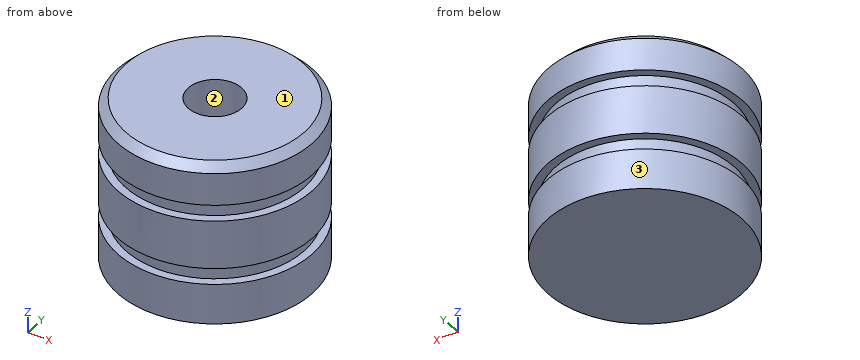
```python
from build123d import *

# Parameters (mm, degrees)
SKETCH1_R                 = 6
BOSS_EXTRUDE1_DEPTH       = 5
CUT_EXTRUDE1_START        = -2.5
SKETCH2_R                 = 6
SKETCH2_R_2               = 5.5
CUT_EXTRUDE1_DEPTH        = 1
CHAMFER1_SIZE             = 0.5
M4X0_7_TAPPED_HOLE1_D     = 3.3
M4X0_7_TAPPED_HOLE1_DEPTH = 8
M4X0_7_TAPPED_HOLE1_TIP   = 0.991420021


with BuildPart() as part:
    # Sketch1 → Boss-Extrude1 (new body, symmetric)
    with BuildSketch(Plane.XY):
        Circle(SKETCH1_R)
    extrude(amount=BOSS_EXTRUDE1_DEPTH, both=True)

    # Sketch2 → Cut-Extrude1 (cut)
    with BuildSketch(Plane.XY.offset(5).offset(CUT_EXTRUDE1_START)):
        Circle(SKETCH2_R)
        Circle(SKETCH2_R_2, mode=Mode.SUBTRACT)
    cut_extrude1 = extrude(amount=-CUT_EXTRUDE1_DEPTH, mode=Mode.SUBTRACT)

    # Mirror1: Cut-Extrude1 across plane
    add(cut_extrude1.mirror(Plane.XY), mode=Mode.SUBTRACT)

    # Chamfer1
    chamfer1_edges = [part.edges().sort_by_distance(p)[0] for p in [
        (-6, 0, 5),
    ]]
    chamfer(chamfer1_edges, length=CHAMFER1_SIZE)

    # M4x0.7 Tapped Hole1
    with Locations(Plane.XY.offset(5)):
        with Locations((0, 0)):
            Hole(M4X0_7_TAPPED_HOLE1_D / 2, depth=M4X0_7_TAPPED_HOLE1_DEPTH)
            with Locations((0, 0, -(M4X0_7_TAPPED_HOLE1_DEPTH + M4X0_7_TAPPED_HOLE1_TIP / 2))):  # 118° drill point
                Cone(0, M4X0_7_TAPPED_HOLE1_D / 2, M4X0_7_TAPPED_HOLE1_TIP, mode=Mode.SUBTRACT)


solid = part.part
```
Could you check a few things on this model? Use its own coordinates, in mm. Face numbers are marked on the shaded views. Round coordinates to 2 decimals unless told otherwise and drop trailing zeros. Loops run counter-clockwise (first coordinate to the right, second up) from the corner with the lowest first, then second, coordinate; pieces in that order, holes last. Notation, with made-up numbers: M 14,84 L 24,84 A13 ccw 24,99 Z; hole C -17,45 d7. An arc over 180 degrees is marked long. Write item = value, one per line.
1. Thinking about a two-plate mould opening in Y: for the marked faces 1, 2 and 3, which applies, +Y half, -Y half, draft (parallel to the pull), parting line (faces both ways), or undercut?
Results below:
face_1 = draft
face_2 = undercut
face_3 = parting line
2. Will these pins go through, and if not, where does the flat tip stop? P1, Ø1, axis at y = -2, z = 0, coming from the +X side; P2, Ø6, axis at x = -4, z = 0.5, coming from the -Y side; P3, Ø1.5, axis at x = -1, z = 0, coming from the +Y side.
Results below:
P1 = 5.81
P2 = -5.92
P3 = 5.99
3. I want a section at A-A, the plane z = -2.75. Write out the boundary of the cut face in (x, y).
Results below:
outline = C 0,0 d12; hole C 0,0 d3.3
4. I need wall thicknesses on probe 1 along Y at (x, z) = (0, 2); probe 2 along Y at (x, z) = (0, -1); probe 3 along X at (y, z) = (-1.5, -0.25). Which ranges of each line are inside material? Lowest first, please.
Results below:
probe_1 = -5.5 to -1.65, 1.65 to 5.5
probe_2 = -6 to -1.65, 1.65 to 6
probe_3 = -5.81 to -0.69, 0.69 to 5.81
